Geometry: final body of the model. Coordinates: model frame, mm. Face numbers are marked on the shaded views. A direction names the side the tool comes from. Give positions to 0.01 mm unless a question says otherwise; leave off trailing zeros. Write each loop counter-clockwise with the first axis right and the second up, starting at its lowest first coordinate (ties: lowest second). Pieces come first, ordered by that corner, then holes. Notation, with made-up numbers: M -30.5,-28 L 14.5,-28 A13 ccw 14.5,-12 Z; hole C 42,42 d5. An arc over 180 degrees is marked long. Use a Markdown table: item, result. Add a question column.
(1) Cut plane A-A (x = -45.5). Output: boundary loops of the cut face in (y, z).
(2) Cut plane D-D (y = 87.5). Output: boundary loops of the cut face in (x, z), plus the area to 3 significant figures.
(3) Draft query along X for the marked faces 3, 4 and 5. Return one class per face: released by +X, released by -X, zero draft, split by the parting line, or undercut.
(4) Reachability of the marked faces 1 and 2 from +Z, -Z, +X, -X, +Y, -Y: full face, straight path, thin tool, end or side. Return the list, or none.
(5) Cut plane C-C (x = -38.5). Output: boundary loops of the cut face in (y, z).
(6) Material intervals for L1, parallel to Z at x = -49.5, y = 82; L2, parallel to Y at x = -36.5, z = 4.8; L3, parallel to X at y = 69.5, z = 4.05, sorted ascending.
(7) Pin query (flat end, axial travel): pin 1 Ø1.5 at (y, z) = (73.5, 1.5) entering from +X; pin 2 Ø3.5 at (x, y) = (-34.25, 70.79) entering from +Z. Return the tip coordinate at first contact, or that it passes through.
(8) Cut plane B-B (z = 0.7). Output: boundary loops of the cut face in (x, y), plus the area to 3 significant figures.
```python
from build123d import *

# Parameters (mm, degrees)
SKETCH1_R           = 20
SKETCH1_R_2         = 1.5
SKETCH1_R_3         = 1
BOSS_EXTRUDE1_DEPTH = 1.5
SKETCH2_R           = 5
SKETCH2_R_2         = 3
BOSS_EXTRUDE2_DEPTH = 4


with BuildPart() as part:
    # Sketch1 → Boss-Extrude1 (new body)
    with BuildSketch(Plane.XY):
        with Locations((-34.248726775, 70.794412983)):
            Circle(SKETCH1_R)
        with Locations((-45.940069726, 77.544412983)):
            Circle(SKETCH1_R_2, mode=Mode.SUBTRACT)
        with Locations((-34.248726775, 84.294412983)):
            Circle(SKETCH1_R_2, mode=Mode.SUBTRACT)
        with Locations((-22.557383823, 77.544412983)):
            Circle(SKETCH1_R_2, mode=Mode.SUBTRACT)
        with Locations((-22.557383823, 64.044412983)):
            Circle(SKETCH1_R_2, mode=Mode.SUBTRACT)
        with Locations((-34.248726775, 57.294412983)):
            Circle(SKETCH1_R_2, mode=Mode.SUBTRACT)
        with Locations((-45.940069726, 64.044412983)):
            Circle(SKETCH1_R_2, mode=Mode.SUBTRACT)
        with Locations((-34.248726775, 70.794412983)):
            Circle(SKETCH1_R_3, mode=Mode.SUBTRACT)
    extrude(amount=BOSS_EXTRUDE1_DEPTH)

    # Sketch2 → Boss-Extrude2 (add)
    with BuildSketch(Plane.XY.offset(1.5)):
        with Locations((-34.248726775, 70.794412983)):
            Circle(SKETCH2_R)
        with Locations((-34.248726775, 70.794412983)):
            Circle(SKETCH2_R_2, mode=Mode.SUBTRACT)
    extrude(amount=BOSS_EXTRUDE2_DEPTH)


solid = part.part
```
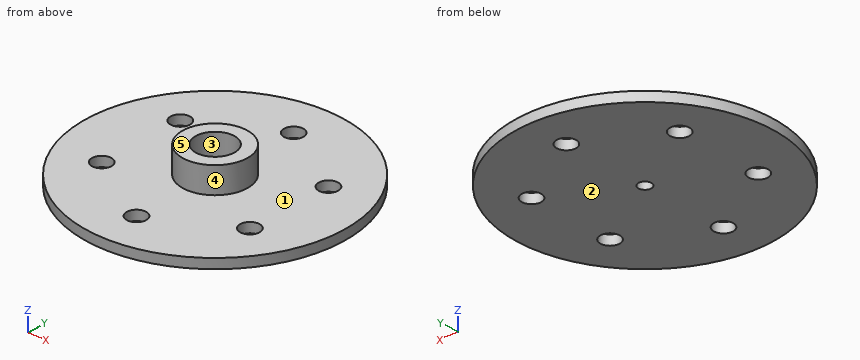
Answer list:
| question | item | result |
|---|---|---|
| 1 | outline | M 54.26,0 L 62.61,0 L 62.61,1.5 L 54.26,1.5 Z; M 65.48,0 L 76.11,0 L 76.11,1.5 L 65.48,1.5 Z; M 78.98,0 L 87.33,0 L 87.33,1.5 L 78.98,1.5 Z |
| 2 | outline | M -45.25,0 L -23.25,0 L -23.25,1.5 L -45.25,1.5 Z |
| 2 | area | 33.0 mm² |
| 3 | face 3 | undercut |
| 3 | face 4 | split by the parting line |
| 3 | face 5 | zero draft |
| 4 | face 1 | +Z |
| 4 | face 2 | -Z, +X, -X, +Y, -Y |
| 5 | outline | M 51.25,0 L 90.34,0 L 90.34,1.5 L 73.43,1.5 L 73.43,5.5 L 68.16,5.5 L 68.16,1.5 L 51.25,1.5 Z |
| 6 | L1 | 0 to 1.5 |
| 6 | L2 | 66.33 to 68.81, 72.78 to 75.26 |
| 6 | L3 | -39.08 to -36.96, -31.54 to -29.42 |
| 7 | pin 1 | x = -14.34 |
| 7 | pin 2 | z = 1.5 |
| 8 | outline | C -34.25,70.79 d40; hole C -45.94,64.04 d3; hole C -45.94,77.54 d3; hole C -34.25,57.29 d3; hole C -34.25,84.29 d3; hole C -34.25,70.79 d2; hole C -22.56,64.04 d3; hole C -22.56,77.54 d3 |
| 8 | area | 1,210 mm² |
